Here's how the part is built. I have some questions about the finished solid (model axes, mm). A direction names the side the tool comes from. Coordinates: 2 decimals unless noted, no trailing zeros. Write each loop counter-clockwise with the first axis right and the second up, starting at its lowest first coordinate (ties: lowest second). Pieces come first, ordered by that corner, then holes.
(1) Please list where these lines run through material, in increasing order: probe 1 along Y at (x, z) = (0, 3.5); probe 2 along Y at (x, z) = (1, 12.25); probe 3 along X at (y, z) = (-9, 9.25).
(2) Imagine slicing it at D-D, the plane y = 6. List the corners of the cut face in (x, z) for me.
(3) For pin 1 Ø4 at (x, z) = (1.5, 6.5) entering from -Y; pin 2 Ø1 at (y, z) = (-19.5, 1.5) entering from +X; pin 3 Ø1 at (y, z) = (9.5, 5) entering from +X, each with a flat end and sliding along its axis, tell me the tip position at first contact or that it passes through.
(4) Thinking about a two-plate mould opening in Y: for faces 1 (the cylindrical face through (-5.506, -24.796, 6.261)), 2 (the flat face through (0, 6, 0)), 3 (the flat face through (0, 5, 6)), 4 (the cylindrical face through (0, -10, 6)), which applies, released by +Y, released by -Y, zero draft, split by the parting line, or undercut?
(5) Imagine slicing it at C-C, the plane z = 8. List the corners of the cut face in (x, y) for me, plus the area to 3 significant figures.
(6) Imagine slicing it at A-A, the plane x = 0. List the corners of the cut face in (y, z) for me, plus the area to 3 significant figures.
(7) Which directions (+Z, -Z, +X, -X, +Y, -Y) give clear straight access to the entire face, cutting with the end or side of a thin tool? Please do faces 5 (the flat face through (-4, 7, 6)), 6 (the flat face through (0, 6, 12.7)).
(8) Imagine slicing it at B-B, the plane y = 0. List the corners of the cut face in (x, z) for me.
```python
from build123d import *

# Parameters (mm, degrees)
SKETCH1_R           = 25.4
BOSS_EXTRUDE1_DEPTH = 12.7


with BuildPart() as part:
    # Sketch1 → Boss-Extrude1 (new body)
    with BuildSketch(Plane.XY):
        Circle(SKETCH1_R)
        with BuildLine():
            Line((-4, 9.16515139), (-4, 5))
            Line((-4, 5), (4, 5))
            Line((4, 5), (4, 9.16515139))
            ThreePointArc((4, 9.16515139), (0, -10), (-4, 9.16515139))
        make_face(mode=Mode.SUBTRACT)
    extrude(amount=BOSS_EXTRUDE1_DEPTH)


solid = part.part
```
Recorded:
1. probe 1: y = -25.4 to -10, 5 to 25.4
1. probe 2: y = -25.38 to -9.95, 5 to 25.38
1. probe 3: x = -23.75 to -4.36, 4.36 to 23.75
2. outline: (-24.68, 0) - (-8, 0) - (-8, 12.7) - (-24.68, 12.7) - close; (-4, 0) - (4, 0) - (4, 12.7) - (-4, 12.7) - close; (8, 0) - (24.68, 0) - (24.68, 12.7) - (8, 12.7) - close
3. pin 1: stops at y = -25.4
3. pin 2: stops at x = 16.86
3. pin 3: stops at x = 23.75
4. face 1: split by the parting line
4. face 2: zero draft
4. face 3: undercut
4. face 4: undercut
5. outline: circle Ø50.8 at (0, 0); hole (-4, 5) - (-4, 9.17) arc R10 ccw (long way) to (4, 9.17) - (4, 5) - close
5. area: 1,750 mm2
6. outline: (-25.4, 0) - (-10, 0) - (-10, 12.7) - (-25.4, 12.7) - close; (5, 0) - (25.4, 0) - (25.4, 12.7) - (5, 12.7) - close
6. area: 455 mm2
7. face 5: +Z, -Z
7. face 6: +Z, +X, -X, +Y, -Y
8. outline: (-25.4, 0) - (-10, 0) - (-10, 12.7) - (-25.4, 12.7) - close; (10, 0) - (25.4, 0) - (25.4, 12.7) - (10, 12.7) - close
